Autodesk Inventor part; units mm, degrees
ref_plane "YZ Plane" through (0, 0, 0) normal (1, 0, 0) x (0, 1, 0)
ref_plane "XZ Plane" through (0, 0, 0) normal (0, 1, 0) x (-1, 0, 0)
ref_plane "XY Plane" through (0, 0, 0) normal (0, 0, 1) x (1, 0, 0)
sketch "Sketch1" plane through (0, 0, 0) normal (0, 1, 0) x (-1, 0, 0)
  line L0 (0, 0) -> (0, -33.655)
  line L1 (0, -33.655) -> (35.687, -33.655)
  line L2 (35.687, -33.655) -> (35.687, 0)
  line L3 (35.687, 0) -> (0, 0)
  line L4 (0, -33.655) -> (2.54, -33.655)
  line L5 (2.54, -33.655) -> (2.54, -30.607)
  circle A0 centre (2.54, -30.607) radius 1.5113
  line L6 (2.54, -30.607) -> (2.54, -7.112)
  circle A1 centre (2.54, -7.112) radius 1.5113
  line L7 (2.54, -7.112) -> (32.004, -7.112)
  circle A2 centre (32.004, -7.112) radius 1.5113
  dimension "d15" = 33.655
  dimension "d16" = 35.687
  dimension "d17" = 2.54
  dimension "d18" = 3.048
  dimension "d19" = 3.0226
  dimension "d20" = 23.495
  dimension "d21" = 29.464
  dimension "d22" = 3.0226
extrude "Extrusion2" add sketch "Sketch1" along normal blind 1.778
properties part number "PCB_model_2"
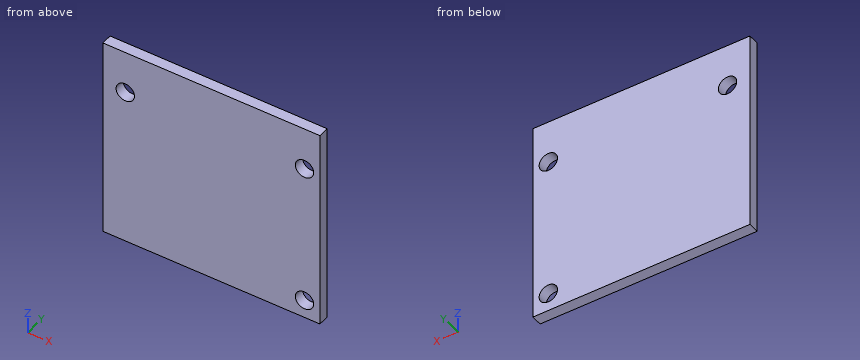
The model under review builds one solid part; all positions refer to its coordinate system, in mm. Round coordinates to 2 decimals unless told otherwise and drop trailing zeros. Write each loop counter-clockwise with the first axis right and the second up, starting at its lowest first coordinate (ties: lowest second). Pieces come first, ordered by that corner, then holes. Notation, with made-up numbers: (29.25, 59) - (64.25, 59) arc R10 cw to (64.25, 73) - close; hole circle Ø3 at (36, -12). An arc over 180 degrees is marked (long way). Answer as CSV lines item,"result". Start each with the question number.
(1) For pin 1 Ø10 at (x, z) = (-30, -16) entering from -Y, flat-tipped, find the tip position at first contact; note if it passes through.
(2) We need section C-C on y = 0.6. State the section outline as (x, z) points (3 decimals).
(3) We need section A-A on x = -2.54. State the section outline as (y, z) points (3 decimals).
(4) We need section B-B on x = -31. State the section outline as (y, z) points (3 decimals), plus the area to 3 significant figures.
(5) To check wall thickness, follow line 1 (Z direction, x = -2.54, y = 0.4) (3 decimals); line 2 (X direction, y = 1.65, z = -7); line 3 (X direction, y = 1.15, z = -8). State the ranges of each line that lie inside material, in increasing order.
Worked answers:
1,pin 1,"y = 0"
2,outline,"(-35.687, -33.655) - (0, -33.655) - (0, 0) - (-35.687, 0) - close; hole circle Ø3.023 at (-32.004, -7.112); hole circle Ø3.023 at (-2.54, -30.607); hole circle Ø3.023 at (-2.54, -7.112)"
3,outline,"(0, -33.655) - (1.778, -33.655) - (1.778, -32.118) - (0, -32.118) - close; (0, -29.096) - (1.778, -29.096) - (1.778, -8.623) - (0, -8.623) - close; (0, -5.601) - (1.778, -5.601) - (1.778, 0) - (0, 0) - close"
4,outline,"(0, -33.655) - (1.778, -33.655) - (1.778, -8.242) - (0, -8.242) - close; (0, -5.982) - (1.778, -5.982) - (1.778, 0) - (0, 0) - close"
4,area,"55.8 mm²"
5,line 1,"-33.655 to -32.118, -29.096 to -8.623, -5.601 to 0"
5,line 2,"-35.69 to -33.51, -30.5 to -4.05, -1.03 to 0"
5,line 3,"-35.69 to -33.23, -30.78 to -3.76, -1.32 to 0"
